```python
from build123d import *

# Parameters (mm, degrees)
BOSS_EXTRUDE1_DEPTH = 5.08
BOSS_EXTRUDE2_DEPTH = 82.55


with BuildPart() as part:
    # Sketch1 → Boss-Extrude1 (new body)
    with BuildSketch(Plane.XY):
        Polygon((0, 0), (-63.5, 0), (-76.2, 21.997045256), (-76.2, 27.077045256), (12.7, 27.077045256), (12.7, 21.997045256), align=None)
    extrude(amount=BOSS_EXTRUDE1_DEPTH)

    # Sketch2 → Boss-Extrude2 (add)
    with BuildSketch(Plane.XY.offset(5.08)):
        Polygon((-76.2, 21.997045256), (-69.85, 27.077045256), (-76.2, 27.077045256), align=None)
        Polygon((12.7, 21.997045256), (12.7, 27.077045256), (6.35, 27.077045256), align=None)
    extrude(amount=BOSS_EXTRUDE2_DEPTH)


solid = part.part
```
Geometry: final body of the model. Coordinates: model frame, mm. A direction names the side the tool comes from. Coordinates: 2 decimals unless noted, no trailing zeros. Loops run counter-clockwise (first coordinate to the right, second up) from the corner with the lowest first, then second, coordinate; pieces in that order, holes last. Notation, with made-up numbers: (80, 32) -> (112, 32) arc R18 cw to (112, 60) -> close; hole circle Ø10 at (-23, 43). An arc over 180 degrees is marked (long way). Use a Markdown table: item, result. Add a question column.
(1) Section query D-D, the plane y = 12. Return loops of the section in (x, z).
(2) Pin query (flat end, axial travel): pin 1 Ø6 at (x, z) = (3, 36.5) entering from +Y; pin 2 Ø10 at (y, z) = (18.5, 37) entering from +X; pin 3 Ø8 at (x, y) = (-35.5, 10.5) entering from +Z. Return the tip coordinate at first contact, or that it passes through.
(3) Section query B-B, the plane y = 23.75. Return loops of the section in (x, z), plus the area to 3 significant figures.
(4) Section query A-A, the plane z = 82.5. Return loops of the section in (x, y).
(5) Section query C-C, the plane x = -15. Return loops of the section in (y, z).
(6) Mould query, pull axis X, two halves, no side actions, for faces 1 (the flat face through (6.439, 11.153, 2.504)), 2 (the flat face through (-73.07, 24.5, 45.78)), 3 (the flat face through (11, 26, 87.63)), 4 (the flat face through (-31, 14, 5.08)). Classes: pulls with the +X half, pulls with the -X half, needs draft (parallel to the pull), parting line crosses it, or undercut.
(7) Line query: line 1 along Z through (x, y) = (-1, 2); line 2 along X through (y, z) = (25.5, 38); line 3 along Y through (x, z) = (8, 44). Output: solid intervals per line, ascending.
(8) Access query for faces 5 (the flat face through (-76.2, 25, 43)), 6 (the flat face through (9.481, 24.573, 45.777)). Directions: +Z, -Z, +X, -X, +Y, -Y. A direction counts if a zero-diameter tool reaches every point of the face in a straight line with its end or side. Return the directions, or none.
Answer:
| question | item | result |
|---|---|---|
| 1 | outline | (-70.43, 0) -> (6.93, 0) -> (6.93, 5.08) -> (-70.43, 5.08) -> close |
| 2 | pin 1 | passes through |
| 2 | pin 2 | stops at x = 12.7 |
| 2 | pin 3 | stops at z = 5.08 |
| 3 | outline | (-76.2, 0) -> (12.7, 0) -> (12.7, 87.63) -> (10.51, 87.63) -> (10.51, 5.08) -> (-74.01, 5.08) -> (-74.01, 87.63) -> (-76.2, 87.63) -> close |
| 3 | area | 813 mm^2 |
| 4 | outline | (-76.2, 22) -> (-69.85, 27.08) -> (-76.2, 27.08) -> close; (6.35, 27.08) -> (12.7, 22) -> (12.7, 27.08) -> close |
| 5 | outline | (0, 0) -> (27.08, 0) -> (27.08, 5.08) -> (0, 5.08) -> close |
| 6 | face 1 | pulls with the +X half |
| 6 | face 2 | undercut |
| 6 | face 3 | needs draft |
| 6 | face 4 | undercut |
| 7 | line 1 | z = 0 to 5.08 |
| 7 | line 2 | x = -76.2 to -71.82, 8.32 to 12.7 |
| 7 | line 3 | y = 25.76 to 27.08 |
| 8 | face 5 | +Z, -Z, -X, +Y, -Y |
| 8 | face 6 | +Z, -Y |
